Part model, mm, in its own coordinate system. A direction names the side the tool comes from. Round coordinates to 2 decimals unless told otherwise and drop trailing zeros. Order: outer loops, then holes, each group sorted by start corner. A loop starts at its lowest first (then second) coordinate and runs counter-clockwise, first axis right, second up. Notation, with made-up numbers: (-20.5, -7) -> (19.5, -7) arc R26 ccw to (19.5, 26) -> close; hole circle Ø5 at (2.5, -29.75). An arc over 180 degrees is marked (long way). Answer as a JSON object with one key per item and string values. Group by question number.
```python
from build123d import *

# Parameters (mm, degrees)
SURFACE_EXTRUDE1_1_DEPTH = 120
THICKEN1_T2              = 15
SKETCH5_W                = 90
SKETCH5_H                = 120
CUT_EXTRUDE1_DEPTH       = 120
SKETCH4_W                = 120
SKETCH4_H                = 400
THICKEN2_T1              = 12
FILLET1_R                = 10
FILLET2_R                = 10
SKETCH6_R                = 5
BOSS_EXTRUDE1_DEPTH      = 40
CHAMFER1_SIZE            = 2
CHAMFER2_SIZE            = 2
SKETCH7_W                = 380
SKETCH7_H                = 120
BOSS_EXTRUDE2_DEPTH      = 40
CUT_EXTRUDE2_DEPTH       = 380
SKETCH9_W                = 3
SKETCH9_H                = 120
CUT_EXTRUDE3_DEPTH       = 440
FILLET4_R                = 2
FILLET5_R                = 2
SKETCH10_W               = 40
SKETCH10_H               = 120
CUT_EXTRUDE4_DEPTH       = 20
SKETCH11_W               = 20
SKETCH11_H               = 120
BOSS_EXTRUDE3_DEPTH      = 10
FILLET6_R                = 10


with BuildPart() as body_1:
    # Surface-Extrude1: a surface, the sketch's curves swept straight by 120 mm
    with BuildLine(Plane(origin=(0, 0, 0), x_dir=(1, 0, 0), z_dir=(0, 1, 0)), mode=Mode.PRIVATE) as surface_extrude1_1_path:
        Line((60, -200), (-60, -200))
        Line((-60, -200), (-60, 200))
        Line((-60, 200), (60, 200))
        Line((60, 200), (60, -200))
    surface_extrude1_1 = Shell.extrude(surface_extrude1_1_path.wire(), (0 * SURFACE_EXTRUDE1_1_DEPTH, 1 * SURFACE_EXTRUDE1_1_DEPTH, 0 * SURFACE_EXTRUDE1_1_DEPTH))
    add(Solid.thicken(surface_extrude1_1, -THICKEN1_T2))

    # Sketch5 → Cut-Extrude1 (cut)
    with BuildSketch(Plane.XY.offset(-185)):
        with Locations((0, 60)):
            Rectangle(SKETCH5_W, SKETCH5_H)
    extrude(amount=-CUT_EXTRUDE1_DEPTH, mode=Mode.SUBTRACT)

    # Sketch4 → Surface-Plane1: a flat surface bounded by the sketch
    with BuildSketch(Plane(origin=(0, 0, 0), x_dir=(1, 0, 0), z_dir=(0, 1, 0)), mode=Mode.PRIVATE) as surface_plane1_2_region:
        Rectangle(SKETCH4_W, SKETCH4_H)
    surface_plane1_2 = surface_plane1_2_region.sketch.faces()[0]
    add(Solid.thicken(surface_plane1_2, THICKEN2_T1))

    # Fillet1
    fillet1_edges = [body_1.edges().sort_by_distance(p)[0] for p in [
        (45, 66, 185),
        (45, 12, -7.5),
        (-45, 66, 185),
        (0, 12, 185),
        (-45, 12, -7.5),
    ]]
    fillet(fillet1_edges, radius=FILLET1_R)

    # Fillet2
    fillet2_edges = [body_1.edges().sort_by_distance(p)[0] for p in [
        (-60, 60, 200),
    ]]
    fillet(fillet2_edges, radius=FILLET2_R)

    # Sketch6 → Boss-Extrude1 (add)
    with BuildSketch(Plane(origin=(0, 0, -200), x_dir=(-1, 0, 0), z_dir=(0, 0, -1))):
        with Locations((-52.5, 100)):
            Circle(SKETCH6_R)
        with Locations((52.5, 100)):
            Circle(SKETCH6_R)
        with Locations((-52.5, 70)):
            Circle(SKETCH6_R)
        with Locations((-52.5, 40)):
            Circle(SKETCH6_R)
        with Locations((-52.5, 10)):
            Circle(SKETCH6_R)
        with Locations((52.5, 70)):
            Circle(SKETCH6_R)
        with Locations((52.5, 40)):
            Circle(SKETCH6_R)
        with Locations((52.5, 10)):
            Circle(SKETCH6_R)
    extrude(amount=BOSS_EXTRUDE1_DEPTH)

    # Chamfer1
    chamfer1_edges = [body_1.edges().sort_by_distance(p)[0] for p in [
        (57.5, 100, -240),
        (57.5, 70, -240),
        (57.5, 40, -240),
        (57.5, 10, -240),
    ]]
    chamfer(chamfer1_edges, length=CHAMFER1_SIZE)

    # Chamfer2
    chamfer2_edges = [body_1.edges().sort_by_distance(p)[0] for p in [
        (-47.5, 100, -240),
        (-47.5, 70, -240),
        (-47.5, 40, -240),
        (-47.5, 10, -240),
    ]]
    chamfer(chamfer2_edges, length=CHAMFER2_SIZE)

    # Sketch7 → Boss-Extrude2 (add)
    with BuildSketch(Plane(origin=(60, 0, 0), x_dir=(0, 0, -1), z_dir=(1, 0, 0))):
        with Locations((10, 60)):
            Rectangle(SKETCH7_W, SKETCH7_H)
    extrude(amount=BOSS_EXTRUDE2_DEPTH)

    # Sketch8 → Cut-Extrude2 (cut)
    with BuildSketch(Plane(origin=(0, 0, -200), x_dir=(-1, 0, 0), z_dir=(0, 0, -1))):
        Polygon((-97, 105), (-100, 105), (-100, 15), (-97, 15), (-85, 15), (-90.773502692, 25), (-85, 25), (-80, 25), (-80, 95), (-85, 95), (-90.773502692, 95), (-85, 105), align=None)
        Polygon((-75, 95), (-80, 95), (-80, 25), (-75, 25), (-69.226497308, 25), (-75, 15), (-67, 15), (-67, 105), (-75, 105), (-69.226497308, 95), align=None)
    extrude(amount=-CUT_EXTRUDE2_DEPTH, mode=Mode.SUBTRACT)

    # Sketch9 → Cut-Extrude3 (cut)
    with BuildSketch(Plane(origin=(0, 0, -200), x_dir=(-1, 0, 0), z_dir=(0, 0, -1))):
        with Locations((-98.5, 60)):
            Rectangle(SKETCH9_W, SKETCH9_H)
    extrude(amount=-CUT_EXTRUDE3_DEPTH, mode=Mode.SUBTRACT)

    # Fillet4
    fillet4_edges = [body_1.edges().sort_by_distance(p)[0] for p in [
        (85, 15, -10),
        (85, 105, -10),
        (75, 105, -10),
        (75, 15, -10),
    ]]
    fillet(fillet4_edges, radius=FILLET4_R)

    # Fillet5
    fillet5_edges = [body_1.edges().sort_by_distance(p)[0] for p in [
        (69.226497308, 25, -10),
        (69.226497308, 95, -10),
    ]]
    fillet(fillet5_edges, radius=FILLET5_R)

    # Sketch10 → Cut-Extrude4 (cut)
    with BuildSketch(Plane.XY.offset(180)):
        with Locations((77, 60)):
            Rectangle(SKETCH10_W, SKETCH10_H)
    extrude(amount=CUT_EXTRUDE4_DEPTH, mode=Mode.SUBTRACT)

    # Sketch11 → Boss-Extrude3 (add)
    with BuildSketch(Plane(origin=(57, 0, 0), x_dir=(0, 0, -1), z_dir=(1, 0, 0))):
        with Locations((-190, 60)):
            Rectangle(SKETCH11_W, SKETCH11_H)
    extrude(amount=BOSS_EXTRUDE3_DEPTH)

    # Fillet6
    fillet6_edges = [body_1.edges().sort_by_distance(p)[0] for p in [
        (8.5, 0, 200),
        (-57.071067812, 0, 197.071067812),
        (-60, 0, -5),
    ]]
    fillet(fillet6_edges, radius=FILLET6_R)


solid = body_1.part
```
Q1. Wall check: line 1 (X direction, y = 108.5, z = -96); line 2 (X direction, y = 48.5, z = -85); line 3 (Y direction, x = 72, z = 108.5). Give the ranges that are in metal, low to high. Write a range as [from, to].
Q2. Which spindle directions (+Z, -Z, +X, -X, +Y, -Y) get a long thin tool onto all of the face, cutting with end or side? Do faces 1 (the cylindrical face through (-41.99, 70.31, 182.15)), 2 (the cylindrical face through (-48.815, 13.379, -218.734)), 3 (the flat face through (93, 105, -13)). Say none if no direction does.
Q3. Band-saw the part on B-B (x = -5). List the corners of the cut face in (y, z), plus the area to 3 significant figures.
Q4. Band-saw the part on A-A (z = -204). List the corners of the cut face in (x, y).
Q5. Two-plate mould, pull along Y, no slides. Class faces 4 (the cylindrical face through (42.15, 15.01, -9.88)), 5 (the flat face through (-45, 70, -10)), 6 (the cylindrical face through (-48.815, 73.379, -218.734)): +Y half, -Y half, draft (parallel to the pull), parting line (faces both ways), or undercut.
Q6. Drop flat-ended pins along their axis: pin 1 Ø12 at (y, z) = (90, -38.5) entering from +X; pin 2 Ø20 at (x, y) = (80.5, 9.5) entering from +Z; pin 3 Ø5 at (x, y) = (-32.5, 79) entering from -Z. Give the stop position or say it passes through.
Completed:
{
 "1": {"line 1": "[-60, -45], [45, 97]", "line 2": "[-60, -45], [45, 67]", "line 3": "[0, 15.05], [20.2, 24.88], [95.12, 99.8], [104.95, 120]"},
 "2": {"face 1": "-Z, +Y", "face 2": "-Z", "face 3": "+Z, -Z, +X"},
 "3": {"outline": "(0, -200) -> (12, -200) -> (12, 175) arc R10 cw to (22, 185) -> (120, 185) -> (120, 200) -> (10, 200) arc R10 ccw to (0, 190) -> close", "area": "6,420 mm2"},
 "4": {"outline": "circle Ø10 at (-52.5, 10); circle Ø10 at (-52.5, 40); circle Ø10 at (-52.5, 70); circle Ø10 at (-52.5, 100); circle Ø10 at (52.5, 10); circle Ø10 at (52.5, 40); circle Ø10 at (52.5, 70); circle Ø10 at (52.5, 100)"},
 "5": {"face 4": "+Y half", "face 5": "draft", "face 6": "undercut"},
 "6": {"pin 1": "x = 90.77", "pin 2": "z = 180", "pin 3": "z = 185"}
}
